Verification items for this drawing (mm, ordinates from the low corner). Give positions to 0.01 mm unless a question says otherwise; leave off trailing zeros. Order: outer loops, then holes, each group sorted by start corner. A loop starts at its lowest first (then second) coordinate and runs counter-clockwise, first axis right, second up. Notation, with made-up numbers: M 55.5,33.5 L 74.5,33.5 A26 cw 74.5,52.5 Z; hole C 67.5,-25 d8. An arc over 180 degrees is marked long. One line per question, with ' | ' between items. Start each with the question number.
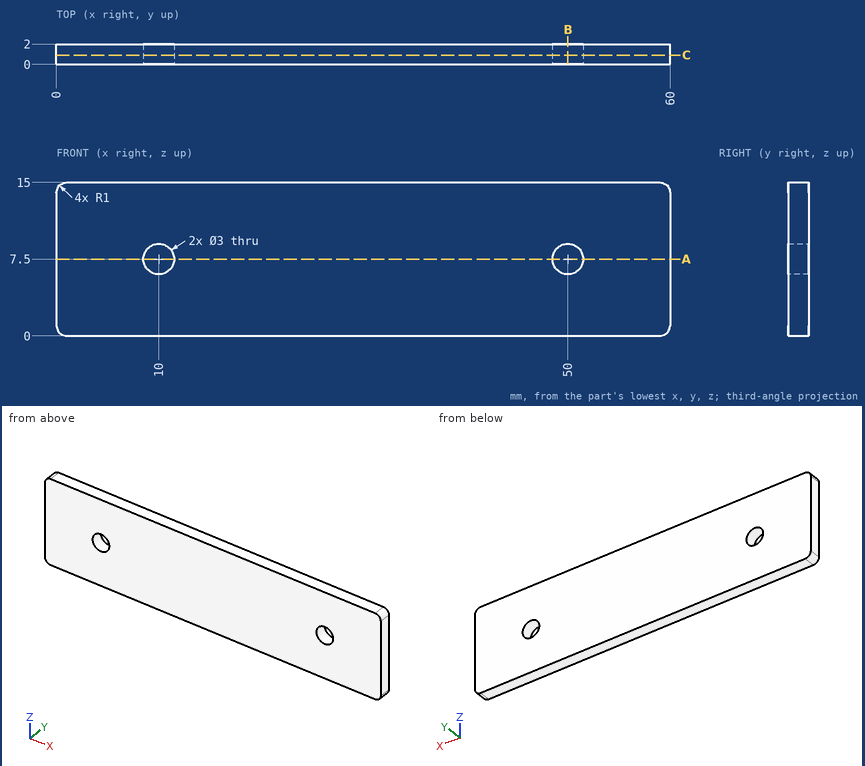
Item 1: Cross-section at C-C, the plane y = 0.9. Record the cut outline in (x, z), plus the area to 3 significant figures.
Item 2: Cross-section at A-A, the plane z = 7.5. Record the cut outline in (x, y), plus the area to 3 significant figures.
Item 3: Cross-section at B-B, the plane x = 50. Record the cut outline in (y, z), plus the area to 3 significant figures.
Item 4: Depth check by flat-ended pin: pin 1 (3 mm diameter, centred on x = 53, z = 3, fed in from -Y). Enter the tip coordinate at first touch or a pass-through.
Item 5: Material ranges on line 1 along X through (y, z) = (0.5, 7.5); line 2 along Z through (x, y) = (50, 0.55), recorded low to high.
Outcome:
1) outline: M 0,1 A1 ccw 1,0 L 59,0 A1 ccw 60,1 L 60,14 A1 ccw 59,15 L 1,15 A1 ccw 0,14 Z; hole C 10,7.5 d3; hole C 50,7.5 d3 | area: 885 mm²
2) outline: M 0,0 L 8.5,0 L 8.5,2 L 0,2 Z; M 11.5,0 L 48.5,0 L 48.5,2 L 11.5,2 Z; M 51.5,0 L 60,0 L 60,2 L 51.5,2 Z | area: 108 mm²
3) outline: M 0,0 L 2,0 L 2,6 L 0,6 Z; M 0,9 L 2,9 L 2,15 L 0,15 Z | area: 24.0 mm²
4) pin 1: stops at y = 0
5) line 1: x = 0 to 8.5, 11.5 to 48.5, 51.5 to 60 | line 2: z = 0 to 6, 9 to 15
